```python
from build123d import *

# Parameters (mm, degrees)
BOSS_EXTRUDE1_DEPTH = 60
SKETCH2_W           = 50
SKETCH2_H           = 5
BOSS_EXTRUDE2_DEPTH = 1


with BuildPart() as part:
    # Sketch1 → Boss-Extrude1 (new body)
    with BuildSketch(Plane.XY):
        Polygon((-25, 0), (25, 0), (25, 5), (26, 5), (26, -1), (10.5, -1), (10.5, -6), (7.5, -6), (7.5, -1), (-7.5, -1), (-7.5, -6), (-10.5, -6), (-10.5, -1), (-26, -1), (-26, 5), (-25, 5), align=None)
    extrude(amount=BOSS_EXTRUDE1_DEPTH)

    # Sketch2 → Boss-Extrude2 (add)
    with BuildSketch(Plane(origin=(0, 0, 0), x_dir=(-1, 0, 0), z_dir=(0, 0, -1))):
        with Locations((0, 2.5)):
            Rectangle(SKETCH2_W, SKETCH2_H)
    extrude(amount=-BOSS_EXTRUDE2_DEPTH)


solid = part.part
```
The model under review builds one solid part; all positions refer to its coordinate system, in mm. A direction names the side the tool comes from. Give positions to 0.01 mm unless a question says otherwise; leave off trailing zeros. Write each loop counter-clockwise with the first axis right and the second up, starting at its lowest first coordinate (ties: lowest second). Pieces come first, ordered by that corner, then holes. Notation, with made-up numbers: (20, 43) - (50, 43) arc R20 cw to (50, 57) - close; hole circle Ø8 at (50.25, -25.75). An arc over 180 degrees is marked (long way). Answer in a Markdown table with one row per item. Add a question column.
1. Wall thickness on line 1 along X through (y, z) = (2, 57); line 2 along X through (y, z) = (-1.25, 8); line 3 along Y through (x, z) = (14, 12.5): over which ranges is each line inside the solid? List them lowest first. Write a range as [from, to].
2. We need section B-B on x = -8.5. Write out the cut boundary in (y, z), then the cut area to 3 significant figures.
3. We need section C-C on y = 3. Write out the cut boundary in (x, z).
4. Insertion check: P1, Ø3, axis at x = -15, y = -2, coming from the +Z side; P2, Ø1.5, axis at x = 2.5, y = 1.5, coming from the +Z side; P3, Ø4, axis at x = 0, z = 50.5, coming from the +Y side; P4, Ø2, axis at y = -4, z = 8.5, coming from the +X side. Each pin has a flat end and moves straight along its axis. Give the tip position at first contact, or say it passes through.
5. Tool access review of faces 4 (the flat face through (0, 3, 1)), 5 (the flat face through (0, -1, 30)), 6 (the flat face through (-10.5, -4, 30)), 7 (the flat face through (18, -1, 30)), 8 (the flat face through (26, 2, 30)): name each direction out of +Z, -Z, +X, -X, +Y, -Y from which nothing blocks a thin tool from reaching the whole face with its end or side.
6. Draft analysis for pull direction X (two halves, no side actions). For faces 1 (the flat face through (7.5, -4, 30)), 2 (the flat face through (-26, 2, 30)), 3 (the flat face through (-9, -6, 30)), state which applies: +X half, -X half, draft (parallel to the pull), parting line (faces both ways), or undercut.
7. We need section A-A on y = -5. Write out the cut boundary in (x, z).
8. We need section D-D on z = 10.5. Write out the cut boundary in (x, y).
Ans:
| question | item | result |
|---|---|---|
| 1 | line 1 | x = [-26, -25], [25, 26] |
| 1 | line 2 | x = [-10.5, -7.5], [7.5, 10.5] |
| 1 | line 3 | y = [-1, 0] |
| 2 | outline | (-6, 0) - (5, 0) - (5, 1) - (0, 1) - (0, 60) - (-6, 60) - close |
| 2 | area | 365 mm^2 |
| 3 | outline | (-26, 0) - (26, 0) - (26, 60) - (25, 60) - (25, 1) - (-25, 1) - (-25, 60) - (-26, 60) - close |
| 4 | P1 | stops at z = 60 |
| 4 | P2 | stops at z = 1 |
| 4 | P3 | stops at y = 0 |
| 4 | P4 | stops at x = 10.5 |
| 5 | face 4 | +Z, +Y |
| 5 | face 5 | +Z, -Z, -Y |
| 5 | face 6 | +Z, -Z, -X, -Y |
| 5 | face 7 | +Z, -Z, +X, -Y |
| 5 | face 8 | +Z, -Z, +X, +Y, -Y |
| 6 | face 1 | undercut |
| 6 | face 2 | -X half |
| 6 | face 3 | draft |
| 7 | outline | (-10.5, 0) - (-7.5, 0) - (-7.5, 60) - (-10.5, 60) - close; (7.5, 0) - (10.5, 0) - (10.5, 60) - (7.5, 60) - close |
| 8 | outline | (-26, -1) - (-10.5, -1) - (-10.5, -6) - (-7.5, -6) - (-7.5, -1) - (7.5, -1) - (7.5, -6) - (10.5, -6) - (10.5, -1) - (26, -1) - (26, 5) - (25, 5) - (25, 0) - (-25, 0) - (-25, 5) - (-26, 5) - close |
